```python
from build123d import *

# Parameters (mm, degrees)
SKETCH1_W           = 40.64
SKETCH1_H           = 26.67
SKETCH1_R           = 2.25
SKETCH1_R_2         = 1.05
SKETCH1_R_3         = 6.35
BOSS_EXTRUDE1_DEPTH = 4
FILLET1_R           = 2.54
CHAMFER1_SIZE       = 0.5


with BuildPart() as part:
    # Sketch1 → Boss-Extrude1 (new body)
    with BuildSketch(Plane.XY):
        Rectangle(SKETCH1_W, SKETCH1_H)
        with Locations((-16.51, 9.525)):
            Circle(SKETCH1_R, mode=Mode.SUBTRACT)
        with Locations((16.51, 9.525)):
            Circle(SKETCH1_R, mode=Mode.SUBTRACT)
        with Locations(Location((16.51, -9.525, 0), (0, 0, 180))):
            Circle(SKETCH1_R, mode=Mode.SUBTRACT)
        with Locations(Location((-16.51, -9.525, 0), (0, 0, 180))):
            Circle(SKETCH1_R, mode=Mode.SUBTRACT)
        with Locations((-9.00049, 5.50037)):
            Circle(SKETCH1_R_2, mode=Mode.SUBTRACT)
        with Locations((9.00049, -5.50037)):
            Circle(SKETCH1_R_2, mode=Mode.SUBTRACT)
        Circle(SKETCH1_R_3, mode=Mode.SUBTRACT)
        with Locations(Location((-9.00049, -5.50037, 0), (0, 0, 180))):
            Circle(SKETCH1_R_2, mode=Mode.SUBTRACT)
        with Locations(Location((9.00049, 5.50037, 0), (0, 0, 180))):
            Circle(SKETCH1_R_2, mode=Mode.SUBTRACT)
    extrude(amount=BOSS_EXTRUDE1_DEPTH)

    # Fillet1
    fillet1_edges = [part.edges().sort_by_distance(p)[0] for p in [
        (-20.32, 13.335, 2),
        (20.32, 13.335, 2),
        (20.32, -13.335, 2),
        (-20.32, -13.335, 2),
    ]]
    fillet(fillet1_edges, radius=FILLET1_R)

    # Chamfer1
    chamfer1_edges = [part.edges().sort_by_distance(p)[0] for p in [
        (7.95049, -5.50037, 4),
        (-10.05049, 5.50037, 4),
        (-7.95049, -5.50037, 4),
        (10.05049, 5.50037, 4),
    ]]
    chamfer(chamfer1_edges, length=CHAMFER1_SIZE)


solid = part.part
```
For this review, take the finished solid that the model builds, in its own axes (mm). Round coordinates to 2 decimals unless told otherwise and drop trailing zeros. Write each loop counter-clockwise with the first axis right and the second up, starting at its lowest first coordinate (ties: lowest second). Pieces come first, ordered by that corner, then holes. Notation, with made-up numbers: (51, 73) -> (80, 73) arc R15 cw to (80, 94) -> close; hole circle Ø4 at (50.5, 78). An arc over 180 degrees is marked (long way). Use one line per item in the form item = value.
1) Take a section at D-D, the plane z = 2.35. Count the separate pieces of the cut face and the enclosed holes in it, and give its area (3 significant figures).
Found:
separate_pieces = 1
enclosed_holes = 9
area = 874 mm2
2) Take a section at C-C, the plane x = 0. Write out the cut boundary in (y, z) (3 decimals).
Found:
outline = (-13.335, 0) -> (-6.35, 0) -> (-6.35, 4) -> (-13.335, 4) -> close; (6.35, 0) -> (13.335, 0) -> (13.335, 4) -> (6.35, 4) -> close
3) Take a section at B-B, the plane x = -16.51. Write out the cut boundary in (y, z) (3 decimals), and give its area (3 significant figures).
Found:
outline = (-13.335, 0) -> (-11.775, 0) -> (-11.775, 4) -> (-13.335, 4) -> close; (-7.275, 0) -> (7.275, 0) -> (7.275, 4) -> (-7.275, 4) -> close; (11.775, 0) -> (13.335, 0) -> (13.335, 4) -> (11.775, 4) -> close
area = 70.7 mm2
4) Take a section at A-A, the plane y = 0. Write out the cut boundary in (x, z), and give its area (3 significant figures).
Found:
outline = (-20.32, 0) -> (-6.35, 0) -> (-6.35, 4) -> (-20.32, 4) -> close; (6.35, 0) -> (20.32, 0) -> (20.32, 4) -> (6.35, 4) -> close
area = 112 mm2
5) To check wall thickness, follow L1, parallel to X at y = 8.25, z = 1.35; L2, parallel to X at y = -10.5, z = 0.45; L3, parallel to Y at x = 16, z = 1.4 (3 decimals). State the ranges of each line that lie inside material, in increasing order. Write a range as from..to.
Found:
L1 = -20.32..-18.36, -14.66..14.66, 18.36..20.32
L2 = -20.32..-18.54, -14.48..14.48, 18.54..20.32
L3 = -13.335..-11.716, -7.334..7.334, 11.716..13.335
6) Mouldability with a two-part tool opening along X and no side actions: class faces 1 (the cylindrical face through (14.364, -10.201, 1.972)), 2 (the flat face through (-20.32, 0, 2)), 3 (the cylindrical face through (19.556, 12.611, 2.028)) as +X half, -X half, draft (parallel to the pull), parting line (faces both ways), or undercut.
Found:
face_1 = undercut
face_2 = -X half
face_3 = +X half
